from build123d import *

# Parameters (mm, degrees)
SKETCH1_W             = 4.8
SKETCH1_H             = 3.15
BOSS_EXTRUDE1_DEPTH   = 40
BOSS_EXTRUDE1_2_DEPTH = 40
SKETCH2_W             = 4.8
SKETCH2_H             = 9
BOSS_EXTRUDE2_DEPTH   = 5
BOSS_EXTRUDE3_DEPTH   = 9
BOSS_EXTRUDE4_DEPTH   = 10
FILLET1_R             = 5
FILLET2_R             = 3
FILLET3_R             = 3


with BuildPart() as part:
    # Sketch1 → Boss-Extrude1 (new body)
    with BuildSketch(Plane(origin=(0, 0, 0), x_dir=(1, 0, 0), z_dir=(0, 1, 0))):
        with Locations((2.4, 7.425)):
            Rectangle(SKETCH1_W, SKETCH1_H)
    extrude(amount=BOSS_EXTRUDE1_DEPTH)



with BuildPart() as body_2:
    # Sketch1 → Boss-Extrude1 2 (new body)
    with BuildSketch(Plane(origin=(0, 0, 0), x_dir=(1, 0, 0), z_dir=(0, 1, 0))):
        with Locations((2.4, 1.575)):
            Rectangle(SKETCH1_W, SKETCH1_H)
    extrude(amount=BOSS_EXTRUDE1_2_DEPTH)


with BuildPart() as part_1:
    add(part.part)

    add(body_2.part)  # Boss-Extrude2 merges body 2
    # Sketch2 → Boss-Extrude2 (add)
    with BuildSketch(Plane.XZ):
        with Locations((2.4, -4.5)):
            Rectangle(SKETCH2_W, SKETCH2_H)
    extrude(amount=BOSS_EXTRUDE2_DEPTH)

    # Sketch3 → Boss-Extrude3 (add)
    with BuildSketch(Plane(origin=(4, 0, 0), x_dir=(-1, 0, 0), z_dir=(0, 0, -1))):
        Polygon((-5.8, -17.071067812), (4, -7.271067812), (4, -5), (-0.8, -5), (-10.8, -15), (-10.8, -18.071067812), (-5.8, -18.071067812), align=None)
    extrude(amount=BOSS_EXTRUDE3_DEPTH)

    # Sketch4 → Boss-Extrude4 (add)
    with BuildSketch(Plane.XZ.offset(18.071067812)):
        with BuildLine():
            Line((9.8, 0), (9.8, -4.5))
            ThreePointArc((9.8, -4.5), (9.94774, -2.230843129), (10.388465475, 0))
            Line((10.388465475, 0), (9.8, 0))
        make_face()
        with BuildLine():
            ThreePointArc((10.388465475, -9), (9.94774, -6.769156871), (9.8, -4.5))
            Line((9.8, -4.5), (9.8, -9))
            Line((9.8, -9), (10.388465475, -9))
        make_face()
        with BuildLine():
            ThreePointArc((21.05, -15.325317547), (16.474682453, -10.75), (14.8, -4.5))
            Line((14.8, -4.5), (14.8, -9))
            Line((14.8, -9), (10.388465475, -9))
            ThreePointArc((10.388465475, -9), (13.407080463, -15.141277495), (18.55, -19.655444566))
            Line((18.55, -19.655444566), (21.05, -15.325317547))
        make_face()
        with BuildLine():
            Line((14.8, -9), (14.8, -4.5))
            Line((14.8, -4.5), (9.8, -4.5))
            ThreePointArc((9.8, -4.5), (9.94774, -6.769156871), (10.388465475, -9))
            Line((10.388465475, -9), (14.8, -9))
        make_face()
        with BuildLine():
            Line((9.8, -4.5), (14.8, -4.5))
            Line((14.8, -4.5), (14.8, 0))
            Line((14.8, 0), (10.388465475, 0))
            ThreePointArc((10.388465475, 0), (9.94774, -2.230843129), (9.8, -4.5))
        make_face()
        with BuildLine():
            Line((14.8, 0), (14.8, -4.5))
            ThreePointArc((14.8, -4.5), (16.474682453, 1.75), (21.05, 6.325317547))
            Line((21.05, 6.325317547), (18.55, 10.655444566))
            ThreePointArc((18.55, 10.655444566), (13.407080463, 6.141277495), (10.388465475, 0))
            Line((10.388465475, 0), (14.8, 0))
        make_face()
    extrude(amount=BOSS_EXTRUDE4_DEPTH)

    # Fillet1
    # the kernel refuses this fillet: 5 mm, written as the material it takes off along each edge
    with BuildSketch(Plane(origin=(16.412896925, 40, -3.15), x_dir=(0, 0, 1), z_dir=(-1, 0, 0))) as fillet1_piece_1:
        with BuildLine():
            CenterArc((5, -4.64515877), FILLET1_R, 111.715617283, 68.284382717)
            Line((0, -4.64515877), (-0.1, -4.64515877))
            Line((-0.1, -4.64515877), (-0.1, 0))
            Line((-0.1, 0), (0, 0.1))
            ThreePointArc((0, 0.1), (1.575, 0.1), (3.113, 0.092903175))
            Line((3.113, 0.092903175), (3.15, 0))
        make_face()
    extrude(amount=28.025793851, mode=Mode.SUBTRACT)
    with BuildSketch(Plane(origin=(-11.612896925, 40, -5.85), x_dir=(0, -1, 0), z_dir=(1, 0, 0))) as fillet1_piece_2:
        with BuildLine():
            CenterArc((4.64515877, 5), FILLET1_R, 201.715617283, 68.284382717)
            Line((0, 3.15), (-0.092903175, 3.113))
            ThreePointArc((-0.092903175, 3.113), (-0.1, 1.575), (-0.1, 0))
            Line((-0.1, 0), (0, -0.1))
            Line((0, -0.1), (4.64515877, -0.1))
            Line((4.64515877, -0.1), (4.64515877, 0))
        make_face()
    extrude(amount=28.025793851, mode=Mode.SUBTRACT)

    # Fillet2
    # the kernel refuses this fillet: 3 mm, written as the material it takes off along each edge
    with BuildSketch(Plane(origin=(21.05, -11.303801998, 6.325317547), x_dir=(-0.8133042312871992, 0, -0.581838660945058), z_dir=(0, -1, 0))) as fillet2_piece_1:
        with BuildLine():
            CenterArc((2.722578478, -2.985784367), FILLET2_R, 95.579968436, 78.840063128)
            Line((-0.263205889, -2.69407953), (0, 0))
            ThreePointArc((0, 0), (1.21543682, -0.059231803), (2.430873641, 0))
        make_face()
    extrude(amount=23.534531629, mode=Mode.SUBTRACT)
    with BuildSketch(Plane(origin=(21.05, -11.303801998, -15.325317547), x_dir=(-0.4999999999999966, 0, -0.8660254037844407), z_dir=(0, -1, 0))) as fillet2_piece_2:
        with BuildLine():
            CenterArc((2.706906326, -3), FILLET2_R, 90, 78.840063128)
            ThreePointArc((-0.236365866, -2.419354839), (-0.059231803, -1.21543682), (0, 0))
            Line((0, 0), (2.706906326, 0))
        make_face()
    extrude(amount=23.534531629, mode=Mode.SUBTRACT)
    with BuildSketch(Plane(origin=(18.55, -8.969979336, -19.655444566), x_dir=(-0.8093218589148085, 0, 0.5873654132502858), z_dir=(0, -1, 0))) as fillet2_piece_3:
        with BuildLine():
            CenterArc((3.328398071, -2.983727989), FILLET2_R, 84.02972802, 101.940543961)
            Line((0.344670082, -3.295765308), (0, 0))
            ThreePointArc((0, 0), (1.820217695, 0.094920065), (3.64043539, 0))
        make_face()
    extrude(amount=28.202176951, mode=Mode.SUBTRACT)
    with BuildSketch(Plane(origin=(18.55, -8.969979336, 10.655444566), x_dir=(-0.8093218589148087, 0, -0.5873654132502856), z_dir=(0, -1, 0))) as fillet2_piece_4:
        with BuildLine():
            CenterArc((3.328398071, 2.983727989), FILLET2_R, 174.02972802, 101.940543961)
            Line((0.344670082, 3.295765308), (0, 0))
            ThreePointArc((0, 0), (1.820217695, -0.094920065), (3.64043539, 0))
        make_face()
    extrude(amount=28.202176951, mode=Mode.SUBTRACT)

    # Fillet3
    fillet3_edges = [part_1.edges().sort_by_distance(p)[0] for p in [
        (4.8, -5, -4.5),
        (9.8, -17.071067812, -4.5),
        (0, -7.271067812, -4.5),
        (14.8, -15, -4.5),
    ]]
    fillet(fillet3_edges, radius=FILLET3_R)


solid = part_1.part
Design review of the part built by this model. Coordinates are the model's own, in mm. A direction names the side the tool comes from. Give positions to 0.01 mm unless a question says otherwise; leave off trailing zeros. Loops run counter-clockwise (first coordinate to the right, second up) from the corner with the lowest first, then second, coordinate; pieces in that order, holes last. Notation, with made-up numbers: M 61.5,35.5 L 86.5,35.5 A12 cw 86.5,45.5 Z; hole C 82.5,8 d10. An arc over 180 degrees is marked long. One line per question, with ' | ' between items. Start each with the question number.
1. Insertion check: P1, Ø8, axis at x = 17, z = -9.5, coming from the +Y side; P2, Ø8, axis at x = 9, y = 21.5, coming from the +Z side; P3, Ø0.5, axis at y = -17.5, z = -2.5, coming from the +X side; P4, Ø1, axis at x = 8.5, z = -3.5, coming from the +Y side. Each pin has a flat end and moves straight along its axis. Give the tip position at first contact, or say it passes through.
2. Add section B-B (z = -2). Write out the cut boundary in (x, y).
3. To check wall thickness, follow L1, parallel to Z at x = 3.25, y = 4.5; L2, parallel to X at y = 18, z = -6.75; L3, parallel to Z at x = 8.5, y = -12. State the ranges of each line that lie inside material, in increasing order.
4. Add section D-D (y = -1). Write out the cut boundary in (x, z).
5. The part is to be moulded in two halves that separate along Z. For faces 6 (the face through (2.37, 38.2, -6.74)), 7 (the face through (0.235, -7.192, -4.563)), 8 (the face through (12.34, -23, -13.58)), 9 (the face through (12.413, -23.001, 4.699)), say which applies: released by +Z, released by -Z, zero draft, split by the parting line, or undercut.
6. Add section A-A (y = 24). Write out the cut boundary in (x, z).
7. For faces 1 (the face through (17.859, -23.001, 9.275)), 2 (the face through (0, 17, -2)), 3 (the face through (9.8, -23, -4)), 4 (the face through (2, 17, -5.85)), 5 (the face through (4.8, 18, -7)), list the 3-axis set-ups (+Z, -Z, +X, -X, +Y, -Y) from which the entire face can be reached by the end or side of a thin tool; tool diameter is ignored.
8. Add section C-C (x = 2.5). Write out the cut boundary in (y, z).
Worked out:
1) P1: stops at y = -13.23 | P2: passes through | P3: stops at x = 14.8 | P4: stops at y = -8.2
2) outline: M 0,-6.03 A3 ccw 0.88,-8.15 L 8.92,-16.19 A3 cw 9.8,-18.31 L 9.8,-28.07 L 15.05,-28.07 L 15.05,-18.07 L 14.8,-18.07 L 14.8,-16.24 A3 ccw 13.92,-14.12 L 5.68,-5.88 A3 cw 4.8,-3.76 L 4.8,38.55 L 0,38.55 Z
3) L1: z = -9 to -5.85, -3.15 to 0 | L2: x = 0 to 4.8 | L3: z = -9 to 0
4) outline: M 0,-9 L 4.8,-9 L 4.8,0 L 0,0 Z
5) face 6: undercut | face 7: zero draft | face 8: released by -Z | face 9: released by +Z
6) outline: M 0,-9 L 4.8,-9 L 4.8,-5.85 L 0,-5.85 Z; M 0,-3.15 L 4.8,-3.15 L 4.8,0 L 0,0 Z
7) face 1: +Z, +Y, -Y | face 2: +Z, -Z, -X, +Y, -Y | face 3: +Z, -Z, -X, -Y | face 4: +X, -X, +Y | face 5: +Z, -Z, +X, +Y
8) outline: M -9.77,-9 L 40,-9 A5 ccw 35.35,-5.85 L 0,-5.85 L 0,-3.15 L 35.35,-3.15 A5 ccw 40,0 L -9.77,0 Z
